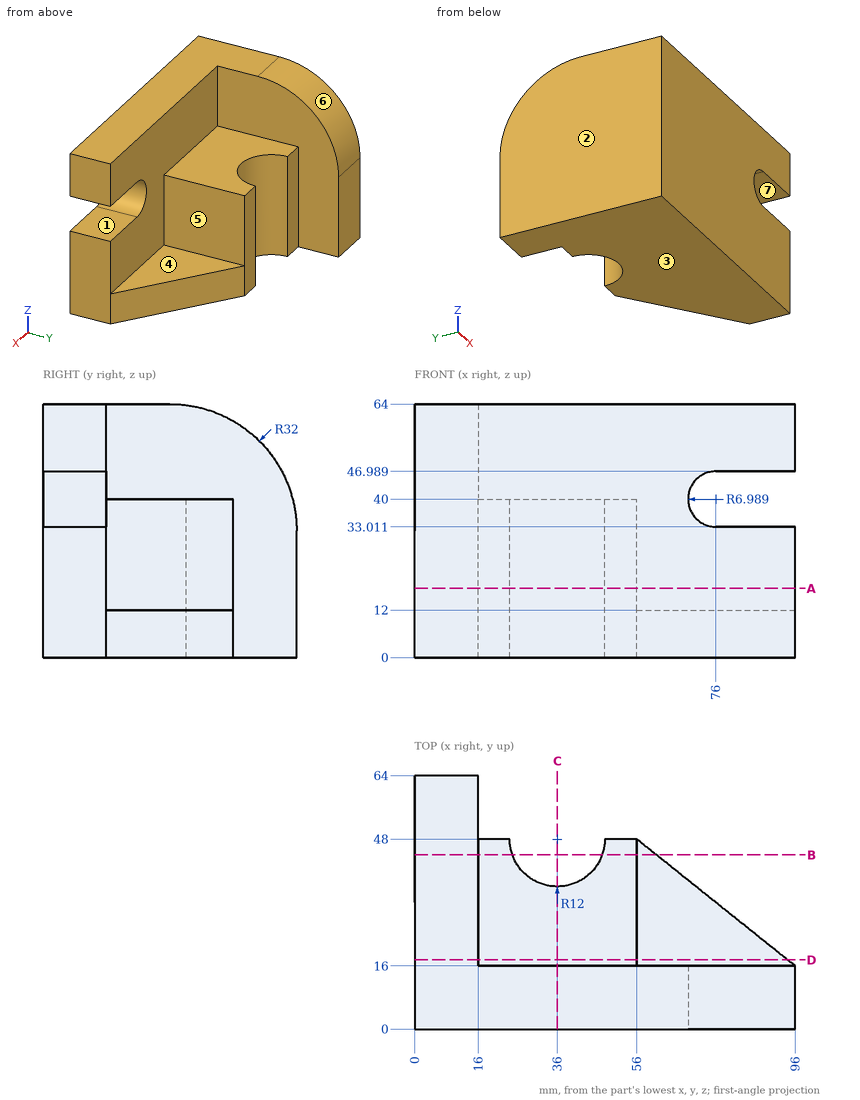
The drawing under review shows one solid part. Ordinate dimensions are in mm from its lowest x, y, z. A direction names the side the tool comes from. Round coordinates to 2 decimals unless told otherwise and drop trailing zeros. Loops run counter-clockwise (first coordinate to the right, second up) from the corner with the lowest first, then second, coordinate; pieces in that order, holes last. Notation, with made-up numbers: (83, 4) - (88, 4) arc R7 cw to (88, 9) - close; hole circle Ø7 at (-34.75, -27.75). An arc over 180 degrees is marked (long way). Put each result on its own line as item: value. Start each with the question number.
1. Consider section B-B on y = 44. State the section outline as (x, z) points, plus the area to 3 significant figures.
2. Consider section D-D on y = 17.5. State the section outline as (x, z) points (3 decimals).
3. Consider section A-A on z = 17.5. State the section outline as (x, y) points, plus the area to 3 significant figures.
4. Insertion check: P1, Ø5, axis at x = 84, y = 9, coming from the -Z side; P2, Ø5, axis at x = 62.5, y = 34.5, coming from the +Z side; P3, Ø4, axis at x = 21, z = 29.5, coming from the +Y side; P4, Ø5, axis at x = 86, z = 29.5, coming from the +Y side. Each pin has a flat end and moves straight along its axis. Give the tip position at first contact, or say it passes through.
5. For probe 1 along Z at (x, y) = (23, 45.5); probe 2 along X at (y, z) = (25.5, 18); probe 3 along Z at (x, y) = (59.5, 37.5), list the stretches that pass through material, from the lowest coordinate up. Write a range as [from, to].
6. For the marked faces 5, 6 and 7, list the 3-axis set-ups (+Z, -Z, +X, -X, +Y, -Y) from which the entire face can be reached by the end or side of a thin tool; tool diameter is ignored.
7. Mouldability with a two-part tool opening along Z and no side actions: class the marked faces 1, 2, 3 and 4 as +Z half, -Z half, draft (parallel to the pull), parting line (faces both ways), or undercut.
8. Consider section C-C on x = 36. State the section outline as (y, z) points, plus the area to 3 significant figures.
Result sheet:
1. outline: (0, 0) - (24.69, 0) - (24.69, 40) - (16, 40) - (16, 61.66) - (0, 61.66) - close; (47.31, 0) - (61, 0) - (61, 12) - (56, 12) - (56, 40) - (47.31, 40) - close
1. area: 1,740 mm^2
2. outline: (0, 0) - (94.125, 0) - (94.125, 12) - (56, 12) - (56, 40) - (16, 40) - (16, 64) - (0, 64) - close
3. outline: (0, 0) - (96, 0) - (96, 16) - (56, 16) - (56, 48) - (48, 48) arc R12 cw to (24, 48) - (16, 48) - (16, 64) - (0, 64) - close
3. area: 3,360 mm^2
4. P1: z = 0
4. P2: z = 12
4. P3: y = 48
4. P4: y = 16
5. probe 1: [0, 40]
5. probe 2: [0, 56]
5. probe 3: [0, 12]
6. face 5: +Z, +X, +Y
6. face 6: +Z, +X, -X, +Y
6. face 7: +X, +Y, -Y
7. face 1: undercut
7. face 2: draft
7. face 3: -Z half
7. face 4: +Z half
8. outline: (0, 0) - (36, 0) - (36, 40) - (16, 40) - (16, 64) - (0, 64) - close
8. area: 1,820 mm^2
